Source: CAD feature listing. Evaluate the final solid. Frame: model axes, mm. Face numbers are marked on the shaded views. A direction names the side the tool comes from. Give positions to 0.01 mm unless a question says otherwise; leave off trailing zeros. Order: outer loops, then holes, each group sorted by start corner. A loop starts at its lowest first (then second) coordinate and runs counter-clockwise, first axis right, second up. Notation, with made-up numbers: M 37.25,57 L 49.25,57 A18 cw 49.25,77 Z; hole C 70.5,72 d1. An arc over 180 degrees is marked long. Use CSV: the item, a comma, the result in double quotes. Start each with the question number.
Item 1: Section query B-B on y = -11.5. Return loops of the section in (x, z).
Item 2: Ray query, probe 1 along Y at (x, z) = (-3.5, 7.5); probe 2 along X at (y, z) = (10, 5); probe 3 along Y at (x, z) = (11.5, 5.6). Return the intervals inside material, ascending. Write a range as from..to.
Item 3: Section query A-A on z = 2. Return loops of the section in (x, y), and give its area (3 significant figures).
Item 4: First-contact query: pin 1 (4 mm diameter, centred on x = 7, z = 3.5, fed in from +Y); pin 2 (5 mm diameter, centred on x = -11.5, y = 11.5, fed in from -Z); pin 3 (2 mm diameter, centred on x = 8.5, z = 2, fed in from -Y) (3 decimals). Flat tips, straight axial feed; report the tip coordinate or a pass-through.
Item 5: Section query C-C on x = 6.25. Return loops of the section in (y, z).
Item 6: Section query D-D on z = 7.5. Count the separate pieces of the cut face and the enclosed holes in it, and give its area (3 significant figures).
Item 7: Pull-direction query (X, two-part tool) for the marked faces 4, 5 and 6; classes: +X half, -X half, draft (parallel to the pull), parting line (faces both ways), or undercut.
Item 8: Access query for the marked faces 1, 2 and 3. Directions: +Z, -Z, +X, -X, +Y, -Y. A direction counts if a zero-diameter tool reaches every point of the face in a straight line with its end or side. Return the directions, or none.
from build123d import *

# Parameters (mm, degrees)
SKETCH1_R               = 13.5
BOSS_EXTRUDE1_DEPTH     = 4
SKETCH2_W               = 30
SKETCH2_H               = 30
BOSS_EXTRUDE2_DEPTH     = 4
FILLET1_R               = 3
CUT_EXTRUDE1_START      = -9
CUT_EXTRUDE1_DEPTH      = 17
MIRROR2_START           = -9
MIRROR2_COPY_1_DEPTH    = 17
SKETCH5_R               = 2
CUT_EXTRUDE2_DEPTH      = 8
MIRROR4_COPY_1_SKETCH_R = 2
MIRROR4_COPY_1_DEPTH    = 8


with BuildPart() as part:
    # Sketch1 → Boss-Extrude1 (new body)
    with BuildSketch(Plane.XY):
        Circle(SKETCH1_R)
    extrude(amount=BOSS_EXTRUDE1_DEPTH)

    # Sketch2 → Boss-Extrude2 (add)
    with BuildSketch(Plane.XY.offset(4)):
        Rectangle(SKETCH2_W, SKETCH2_H)
    extrude(amount=BOSS_EXTRUDE2_DEPTH)

    # Fillet1
    fillet1_edges = [part.edges().sort_by_distance(p)[0] for p in [
        (15, -15, 6),
        (15, 15, 6),
        (-15, 15, 6),
        (-15, -15, 6),
    ]]
    fillet(fillet1_edges, radius=FILLET1_R)

    # Sketch4 → Cut-Extrude1 (cut)
    with BuildSketch(Plane(origin=(0, 0, 0), x_dir=(-1, 0, 0), z_dir=(0, 0, -1)).offset(CUT_EXTRUDE1_START)):
        with BuildLine():
            Line((-12.459935794, 1), (-1, 1))
            Line((-1, 1), (-1, 12.459935794))
            ThreePointArc((-1, 12.459935794), (-8.838834765, 8.838834765), (-12.459935794, 1))
        make_face()
    cut_extrude1 = extrude(amount=CUT_EXTRUDE1_DEPTH, mode=Mode.SUBTRACT)

    # Mirror1: Cut-Extrude1 across plane
    add(cut_extrude1.mirror(Plane(origin=(0, 0, 0), x_dir=(0, 0, 1), z_dir=(1, 0, 0))), mode=Mode.SUBTRACT)

    # Mirror2: Cut-Extrude1 across plane
    add(cut_extrude1.mirror(Plane.ZX), mode=Mode.SUBTRACT)

    # Mirror2 copy 1 sketch → Mirror2 copy 1 (cut)
    with BuildSketch(Plane(origin=(0, 0, 0), x_dir=(1, 0, 0), z_dir=(0, 0, -1)).offset(MIRROR2_START)):
        with BuildLine():
            Line((-12.459935794, 1), (-1, 1))
            Line((-1, 1), (-1, 12.459935794))
            ThreePointArc((-1, 12.459935794), (-8.838834765, 8.838834765), (-12.459935794, 1))
        make_face()
    extrude(amount=MIRROR2_COPY_1_DEPTH, mode=Mode.SUBTRACT)

    # Sketch5 → Cut-Extrude2 (cut)
    with BuildSketch(Plane(origin=(0, 0, 4), x_dir=(-1, 0, 0), z_dir=(0, 0, -1))):
        with Locations((-11.5, 11.5)):
            Circle(SKETCH5_R)
    cut_extrude2 = extrude(amount=-CUT_EXTRUDE2_DEPTH, mode=Mode.SUBTRACT)

    # Mirror3: Cut-Extrude2 across plane
    add(cut_extrude2.mirror(Plane.ZX), mode=Mode.SUBTRACT)

    # Mirror4: Cut-Extrude2 across plane
    add(cut_extrude2.mirror(Plane(origin=(0, 0, 0), x_dir=(0, 0, 1), z_dir=(1, 0, 0))), mode=Mode.SUBTRACT)

    # Mirror4 copy 1 sketch → Mirror4 copy 1 (cut)
    with BuildSketch(Plane(origin=(0, 0, 4), x_dir=(1, 0, 0), z_dir=(0, 0, -1))):
        with Locations((-11.5, 11.5)):
            Circle(MIRROR4_COPY_1_SKETCH_R)
    extrude(amount=-MIRROR4_COPY_1_DEPTH, mode=Mode.SUBTRACT)


solid = part.part
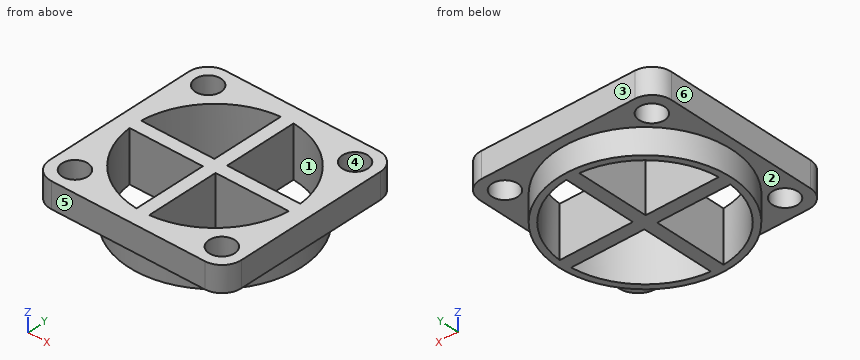
Verdict:
1,outline,"M -15,4 L -13.5,4 L -13.5,8 L -15,8 Z; M -9.5,4 L -7.07,4 L -7.07,0 L -4.9,0 L -4.9,8 L -9.5,8 Z; M -1,0 L 1,0 L 1,8 L -1,8 Z; M 4.9,0 L 7.07,0 L 7.07,4 L 9.5,4 L 9.5,8 L 4.9,8 Z; M 13.5,4 L 15,4 L 15,8 L 13.5,8 Z"
2,probe 1,"-15..-12, -1..1, 12..15"
2,probe 2,"-15..-12.82, -10.18..-7.5, -1..1, 7.5..10.18, 12.82..15"
2,probe 3,"-15..-13.5, -9.5..-4.9, -1..1, 4.9..9.5, 13.5..15"
3,outline,"C 0,0 d27; hole M -12.46,-1 A12.5 ccw -1,-12.46 L -1,-1 Z; hole M -12.46,1 L -1,1 L -1,12.46 A12.5 ccw Z; hole M 1,-12.46 A12.5 ccw 12.46,-1 L 1,-1 Z; hole M 1,1 L 12.46,1 A12.5 ccw 1,12.46 Z"
3,area,"178 mm2"
4,pin 1,"y = 15"
4,pin 2,"z = 4"
4,pin 3,"y = -11.225"
5,outline,"M -15,4 L -11.97,4 L -11.97,0 L -10.83,0 L -10.83,8 L -15,8 Z; M -1,0 L 1,0 L 1,8 L -1,8 Z; M 10.83,0 L 11.97,0 L 11.97,4 L 15,4 L 15,8 L 10.83,8 Z"
6,separate pieces,"1"
6,enclosed holes,"8"
6,area,"447 mm2"
7,face 4,"undercut"
7,face 5,"draft"
7,face 6,"-X half"
8,face 1,"+Z, -Z"
8,face 2,"-Z"
8,face 3,"+Z, -Z, +X, -X, +Y"
